Here's how the part is built. I have some questions about the finished solid (model axes, mm). A direction names the side the tool comes from. Give positions to 0.01 mm unless a question says otherwise; leave off trailing zeros. Loops run counter-clockwise (first coordinate to the right, second up) from the corner with the lowest first, then second, coordinate; pieces in that order, holes last.
Q1. Suppose I cut it at B-B (z = 33.5). List the corners of the cut face in (x, y) for me.
Q2. For faces 1 (the face through (150, -1, 38)), 2 (the face through (-9, 275, 20)), which set-ups out of +Z, -Z, +X, -X, +Y, -Y let a thin tool reach every point of the face, with its end or its side?
Q3. I'm going to push a flat-ended pin straight in: P1, Ø1, axis at y = -16.5, z = 43.5, coming from the -X side. Where does the tip first touch, or does it pass through?
Q4. Suppose I cut it at C-C (x = 23). List the corners of the cut face in (y, z) for me, and give its area (3 significant figures).
Q5. Suppose I cut it at A-A (y = -83). List the corners of the cut face in (x, z) for me.
Q6. I need wall thicknesses on probe 1 along Y at (x, z) = (90, 31.5); probe 2 along X at (y, z) = (65.5, 27); probe 3 along X at (y, z) = (166, 8.5). Which ranges of each line are inside material? Lowest first, please.
Q7. Thinking about a two-plate mould opening in X: for faces 3 (the face through (275, -4, 25)), 4 (the face through (-150, -1, 38)), 5 (the face through (-275, 1, 25)), 6 (the face through (-4, 121, 50)), which applies, pulls with the +X half, pulls with the -X half, needs draft (parallel to the pull), parting line crosses it, or undercut?
```python
from build123d import *

# Parameters (mm, degrees)
F0_W     = 550
F0_H     = 550
F1_DEPTH = 50
F2_R     = 10
F3_W     = 300
F3_H     = 200
F4_DEPTH = 25


with BuildPart() as f1:
    # F0 (on Top) → F1 (new body)
    with BuildSketch(Plane.XY):
        Rectangle(F0_W, F0_H)
    extrude(amount=F1_DEPTH)

    # F2
    f2_edges = [f1.edges().sort_by_distance(p)[0] for p in [
        (-275, 0, 50),
        (0, -275, 50),
        (275, 0, 0),
        (275, -275, 25),
        (275, 275, 25),
        (275, 0, 50),
        (0, 275, 50),
        (0, -275, 0),
        (-275, -275, 25),
        (-275, 0, 0),
    ]]
    fillet(f2_edges, radius=F2_R)

    # F3 (on face) → F4 (cut)
    with BuildSketch(Plane.XY.offset(50)):
        Rectangle(F3_W, F3_H)
    extrude(amount=-F4_DEPTH, mode=Mode.SUBTRACT)


solid = f1.part
```
Solutions:
1. outline: (-275, -265) arc R10 ccw to (-265, -275) - (265, -275) arc R10 ccw to (275, -265) - (275, 265) arc R10 ccw to (265, 275) - (-275, 275) - close; hole (-150, -100) - (150, -100) - (150, 100) - (-150, 100) - close
2. face 1: +Z
2. face 2: +Z, -Z, +X, -X, +Y
3. P1: stops at x = -274.54
4. outline: (-275, 10) arc R10 ccw to (-265, 0) - (275, 0) - (275, 40) arc R10 ccw to (265, 50) - (100, 50) - (100, 25) - (-100, 25) - (-100, 50) - (-265, 50) arc R10 ccw to (-275, 40) - close
4. area: 22,400 mm2
5. outline: (-275, 10) arc R10 ccw to (-265, 0) - (265, 0) arc R10 ccw to (275, 10) - (275, 40) arc R10 ccw to (265, 50) - (150, 50) - (150, 25) - (-150, 25) - (-150, 50) - (-265, 50) arc R10 ccw to (-275, 40) - close
6. probe 1: y = -275 to -100, 100 to 275
6. probe 2: x = -275 to -150, 150 to 275
6. probe 3: x = -274.89 to 274.89
7. face 3: pulls with the +X half
7. face 4: undercut
7. face 5: pulls with the -X half
7. face 6: needs draft
